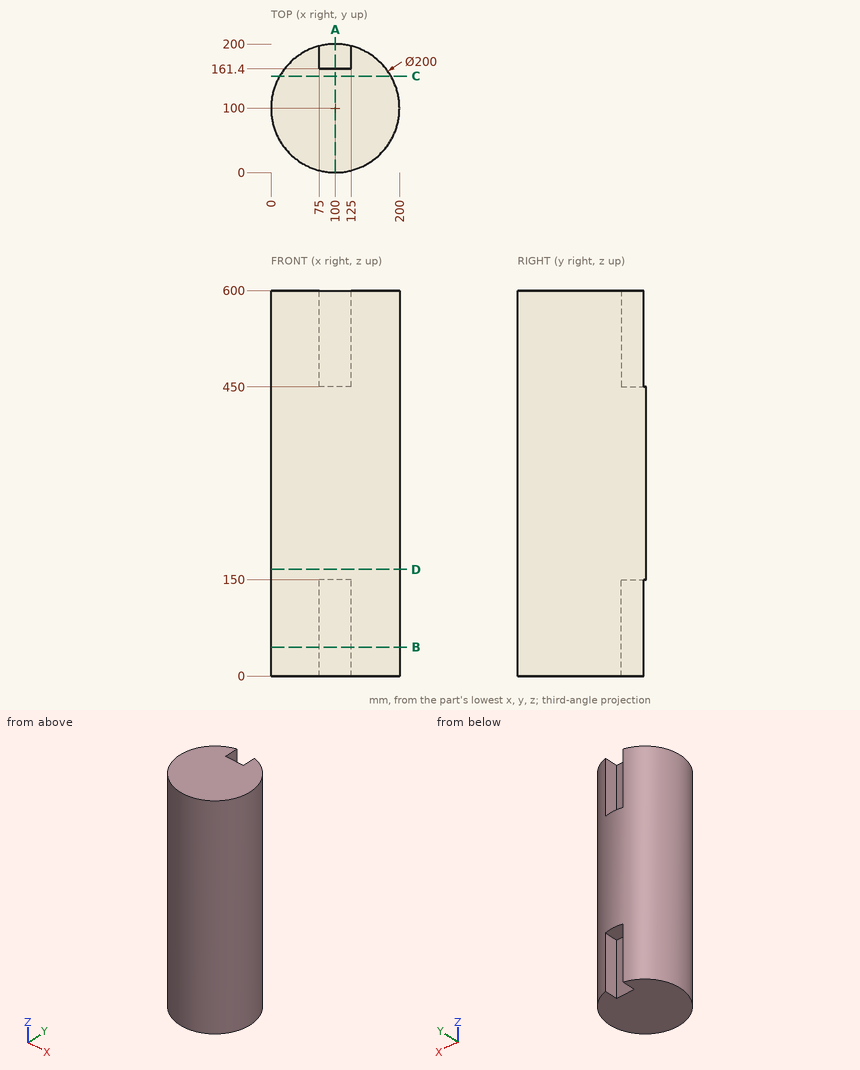
Geometry check sheet. Reference: drawing and pictorial views, mm from the part's lowest x, y, z. Round coordinates to 2 decimals unless told otherwise and drop trailing zeros. Loops run counter-clockwise (first coordinate to the right, second up) from the corner with the lowest first, then second, coordinate; pieces in that order, holes last. Notation, with made-up numbers: M 5,30 L 34,30 A21 cw 34,44 Z; hole C -36,2.25 d1. An arc over 180 degrees is marked long. One line per item, written item: value.
(1) Sectioned sample at D-D, the plane z = 166. Record the cut outline in (x, y).
Computed values:
outline: C 100,100 d200
(2) Thickness scan on line 1 (Z direction, x = 90.5, y = 170); line 2 (Y direction, x = 83, z = 541.5); line 3 (Y direction, x = 48.5, z = 32). Record the ranges inside material, lowest first.
Computed values:
line 1: z = 150 to 450
line 2: y = 1.46 to 161.4
line 3: y = 14.28 to 185.72
(3) Depth check by flat-ended pin: pin 1 Ø10.5 at (y, z) = (185.5, 99.5) entering from -X; pin 2 Ø10 at (y, z) = (24.5, 78) entering from +X; pin 3 Ø1 at (y, z) = (165.5, 421.5) entering from -X. Enter the tip coordinate at first touch or a pass-through.
Computed values:
pin 1: stops at x = 40.33
pin 2: stops at x = 170.92
pin 3: stops at x = 24.01
(4) Sectioned sample at A-A, the plane x = 100. Record the cut outline in (y, z).
Computed values:
outline: M 0,0 L 161.4,0 L 161.4,150 L 200,150 L 200,450 L 161.4,450 L 161.4,600 L 0,600 Z
(5) Sectioned sample at B-B, the plane z = 45. Record the cut outline in (x, y).
Computed values:
outline: M 75,161.4 L 75,196.82 A100 ccw long 125,196.82 L 125,161.4 Z
(6) Sectioned sample at C-C, the plane y = 150. Record the cut outline in (x, z), then the cut area to 3 significant figures.
Computed values:
outline: M 13.4,0 L 186.6,0 L 186.6,600 L 13.4,600 Z
area: 104,000 mm^2
